Answer from the drawing. Dimensions are ordinates in mm from the lowest x, y and z of the part. A direction names the side the tool comes from. Give positions to 0.01 mm unless a question says otherwise; leave off trailing zeros. Order: outer loops, then holes, each group sorted by start corner. A loop starts at its lowest first (then second) coordinate and runs counter-clockwise, first axis right, second up. Notation, with made-up numbers: (-6, 25.25) - (26, 25.25) arc R21 cw to (26, 36.25) - close; hole circle Ø10 at (3, 24.25). An arc over 180 degrees is marked (long way). Write each question's results on one line, items separated by ' | '.
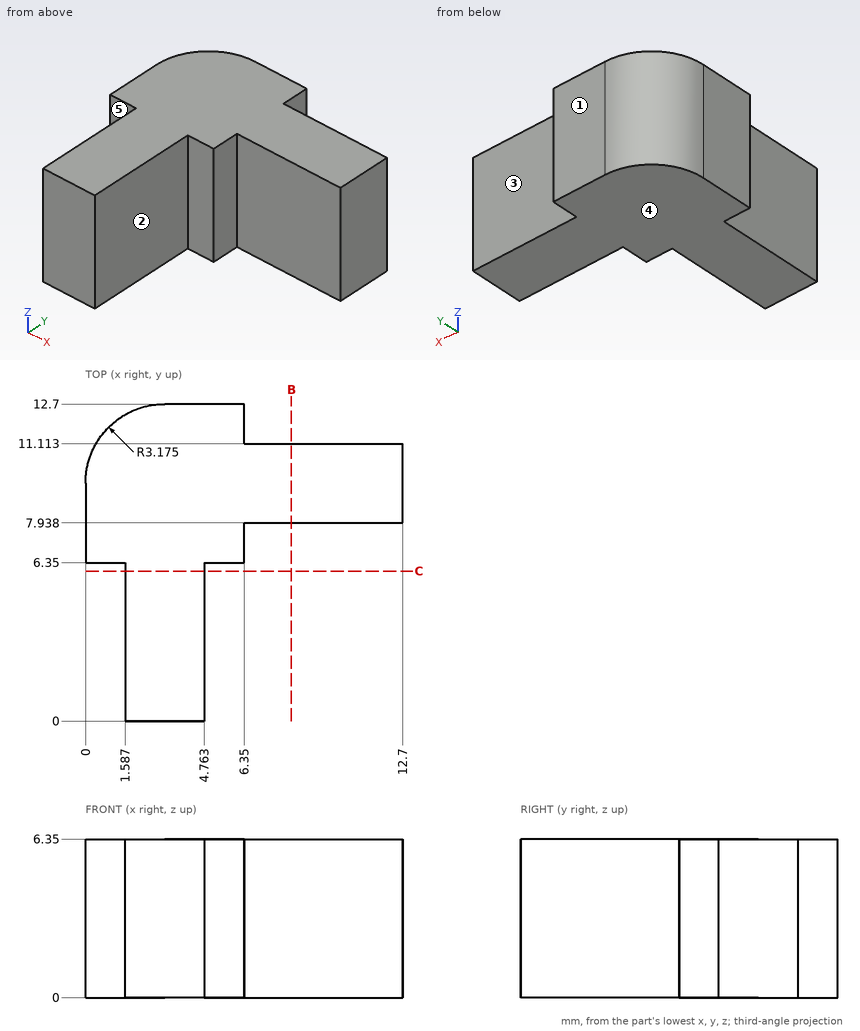
(1) Consider probe 1 along Y at (x, z) = (7.5, 4); probe 2 along X at (y, z) = (1.5, 1.5); probe 3 along Y at (x, z) = (2.75, 5.5). Determine where each line is inside the solid, lowest interval first. Write a range as [from, to].
Conclusion:
probe 1: [7.94, 11.11] | probe 2: [1.59, 4.76] | probe 3: [0, 12.67]
(2) Section B-B (x = 8.25) is taken. Give the vertices of the cut face in (y, z).
Conclusion:
outline: (7.94, 0) - (11.11, 0) - (11.11, 6.35) - (7.94, 6.35) - close
(3) For the marked faces 1, 2, 3, 4 and 5, determine the directions among +Z, -Z, +X, -X, +Y, -Y from which every point of the face is accessible in a straight line to the end or side of a thin tool.
Conclusion:
face 1: +Z, -Z, +X, -X, +Y | face 2: +Z, -Z, +X, -Y | face 3: +Z, -Z, +X, +Y | face 4: -Z, +X, -X, +Y, -Y | face 5: +Z, -Z, -X, -Y
(4) Section C-C (y = 6) is taken. Give the vertices of the cut face in (x, z).
Conclusion:
outline: (1.59, 0) - (4.76, 0) - (4.76, 6.35) - (1.59, 6.35) - close
(5) Each of these flat-tipped pins is pushed along its axis until it touches: pin 1 (1.3 mm diameter, centred on y = 7, z = 1.5, fed in from +X); pin 2 (3 mm diameter, centred on y = 2.5, z = 4, fed in from +X); pin 3 (3 mm diameter, centred on y = 4, z = 2, fed in from -X). Where does it stop, or does it pass through?
Conclusion:
pin 1: x = 6.35 | pin 2: x = 4.76 | pin 3: x = 1.59
